from build123d import *

# Parameters (mm, degrees)
SKETCH1_W                = 170
SKETCH1_H                = 100
BOSS_EXTRUDE1_DEPTH      = 15
SKETCH2_W                = 70
SKETCH2_H                = 70
CUT_EXTRUDE1_DEPTH       = 13
SKETCH3_W                = 70
SKETCH3_H                = 90
CUT_EXTRUDE2_DEPTH       = 12
SKETCH8_W                = 15
SKETCH8_H                = 15
CUT_EXTRUDE9_DEPTH       = 2.5
SKETCH9_W                = 15
SKETCH9_H                = 15
CUT_EXTRUDE10_DEPTH      = 2.5
SKETCH10_W               = 12
SKETCH10_H               = 90
CUT_EXTRUDE11_DEPTH      = 10
SKETCH11_W               = 80
SKETCH11_H               = 90
BOSS_EXTRUDE2_DEPTH      = 10
SKETCH12_W               = 22
SKETCH12_H               = 90
BOSS_EXTRUDE4_DEPTH      = 4
SKETCH2_2_W              = 70
SKETCH2_2_H              = 70
CUT_EXTRUDE12_DEPTH      = 22
SKETCH13_W               = 74
SKETCH13_H               = 74
SKETCH13_W_2             = 70
SKETCH13_H_2             = 70
CUT_EXTRUDE13_DEPTH      = 4
BOSS_EXTRUDE6_DEPTH      = 100
SKETCH15_W               = 5
SKETCH15_H               = 3
CUT_EXTRUDE14_DEPTH      = 15
SKETCH16_R               = 4
SKETCH16_R_2             = 3
BOSS_EXTRUDE7_DEPTH      = 15
SKETCH16_3_R             = 3
CUT_EXTRUDE15_DEPTH      = 15
FILLET1_R                = 2
CUT_EXTRUDE16_DEPTH      = 145.387791679
CUT_EXTRUDE16_DEPTH_BACK = 15


with BuildPart() as part:
    # Sketch1 → Boss-Extrude1 (new body)
    with BuildSketch(Plane.XY):
        with Locations((-16.108033241, 2.077562327)):
            Rectangle(SKETCH1_W, SKETCH1_H)
    extrude(amount=BOSS_EXTRUDE1_DEPTH)

    # Sketch2 → Cut-Extrude1 (cut)
    with BuildSketch(Plane(origin=(0, 0, 0), x_dir=(-1, 0, 0), z_dir=(0, 0, -1))):
        with Locations((-23.891966759, 2.077562327)):
            Rectangle(SKETCH2_W, SKETCH2_H)
    extrude(amount=-CUT_EXTRUDE1_DEPTH, mode=Mode.SUBTRACT)

    # Sketch3 → Cut-Extrude2 (cut)
    with BuildSketch(Plane.XY.offset(15)):
        with Locations((-56.108033241, 2.077562327)):
            Rectangle(SKETCH3_W, SKETCH3_H)
    extrude(amount=-CUT_EXTRUDE2_DEPTH, mode=Mode.SUBTRACT)

    # Sketch8 → Cut-Extrude9 (cut)
    with BuildSketch(Plane(origin=(0, 52.077562327, 0), x_dir=(1, 0, 0), z_dir=(0, 1, 0))):
        with Locations((-93.608033241, -7.5)):
            Rectangle(SKETCH8_W, SKETCH8_H)
    extrude(amount=-CUT_EXTRUDE9_DEPTH, mode=Mode.SUBTRACT)

    # Sketch9 → Cut-Extrude10 (cut)
    with BuildSketch(Plane.XZ.offset(47.922437673)):
        with Locations((-93.608033241, 7.5)):
            Rectangle(SKETCH9_W, SKETCH9_H)
    extrude(amount=-CUT_EXTRUDE10_DEPTH, mode=Mode.SUBTRACT)

    # Sketch10 → Cut-Extrude11 (cut)
    with BuildSketch(Plane.ZY.offset(21.108033241)):
        with Locations((9, 2.077562327)):
            Rectangle(SKETCH10_W, SKETCH10_H)
    extrude(amount=-CUT_EXTRUDE11_DEPTH, mode=Mode.SUBTRACT)

    # Sketch11 → Boss-Extrude2 (add)
    with BuildSketch(Plane.XY.offset(15)):
        Polygon((-86.108033241, -45.422437673), (-86.108033241, -47.922437673), (68.891966759, -47.922437673), (68.891966759, 52.077562327), (-86.108033241, 52.077562327), (-86.108033241, 49.577562327), (-101.108033241, 49.577562327), (-101.108033241, -45.422437673), align=None)
        with Locations((-51.108033241, 2.077562327)):
            Rectangle(SKETCH11_W, SKETCH11_H, mode=Mode.SUBTRACT)
    extrude(amount=BOSS_EXTRUDE2_DEPTH)

    # Sketch12 → Boss-Extrude4 (add)
    with BuildSketch(Plane.ZY.offset(11.108033241)):
        with Locations((14, 2.077562327)):
            Rectangle(SKETCH12_W, SKETCH12_H)
    extrude(amount=BOSS_EXTRUDE4_DEPTH)

    # Sketch2<2> → Cut-Extrude12 (cut)
    with BuildSketch(Plane(origin=(0, 0, 0), x_dir=(-1, 0, 0), z_dir=(0, 0, -1))):
        with Locations((-23.891966759, 2.077562327)):
            Rectangle(SKETCH2_2_W, SKETCH2_2_H)
    extrude(amount=-CUT_EXTRUDE12_DEPTH, mode=Mode.SUBTRACT)

    # Sketch13 → Cut-Extrude13 (cut)
    with BuildSketch(Plane(origin=(0, 0, 0), x_dir=(-1, 0, 0), z_dir=(0, 0, -1))):
        with Locations((-23.891966759, 2.077562327)):
            Rectangle(SKETCH13_W, SKETCH13_H)
        with Locations((-23.891966759, 2.077562327)):
            Rectangle(SKETCH13_W_2, SKETCH13_H_2, mode=Mode.SUBTRACT)
    extrude(amount=-CUT_EXTRUDE13_DEPTH, mode=Mode.SUBTRACT)

    # Sketch14 → Boss-Extrude6 (add)
    with BuildSketch(Plane(origin=(0, 52.077562327, 0), x_dir=(1, 0, 0), z_dir=(0, 1, 0))):
        Polygon((-86.108033241, 0), (-78.108033241, 0), (-86.108033241, 8), align=None)
    extrude(amount=-BOSS_EXTRUDE6_DEPTH)

    # Sketch15 → Cut-Extrude14 (cut)
    with BuildSketch(Plane.ZY.offset(101.108033241)):
        with Locations((12.5, 48.077562327)):
            Rectangle(SKETCH15_W, SKETCH15_H)
        with Locations((12.5, -43.922437673)):
            Rectangle(SKETCH15_W, SKETCH15_H)
    extrude(amount=-CUT_EXTRUDE14_DEPTH, mode=Mode.SUBTRACT)

    # Sketch16 → Boss-Extrude7 (add)
    with BuildSketch(Plane(origin=(-11.108033241, 0, 0), x_dir=(0, 0, -1), z_dir=(1, 0, 0))):
        with Locations(Location((-15.920102605, 0, 0), (0, 0, 90))):
            Circle(SKETCH16_R)
        with Locations(Location((-15.920102605, 0, 0), (0, 0, 90))):
            Circle(SKETCH16_R_2, mode=Mode.SUBTRACT)
    extrude(amount=-BOSS_EXTRUDE7_DEPTH)

    # Sketch16<3> → Cut-Extrude15 (cut)
    with BuildSketch(Plane(origin=(-11.108033241, 0, 0), x_dir=(0, 0, -1), z_dir=(1, 0, 0))):
        with Locations(Location((-15.920102605, 0, 0), (0, 0, 90))):
            Circle(SKETCH16_3_R)
    extrude(amount=-CUT_EXTRUDE15_DEPTH, mode=Mode.SUBTRACT)

    # Fillet1
    # the kernel refuses this fillet: 2 mm, written as the material it takes off along each edge
    with BuildSketch(Plane(origin=(-26.108033241, 0, 15.920102605), x_dir=(0, 1, 0), z_dir=(0, 0, -1))) as fillet1_piece_1:
        with BuildLine():
            CenterArc((2, 1.732050808), FILLET1_R, 300, 60)
            Line((3, 0), (3.02, -0.034641016))
            ThreePointArc((3.02, -0.034641016), (3.5, -0.04), (4, -0.04))
            Line((4, -0.04), (4.04, 0))
            Line((4.04, 0), (4.04, 1.732050808))
            Line((4.04, 1.732050808), (4, 1.732050808))
        make_face()
    revolve(axis=Axis((-26.108033241, 0, 15.920102605), (1, 0, 0)), mode=Mode.SUBTRACT)

    # Sketch17 → Cut-Extrude16 (cut, two sides: drawn at the far end of the back side and taken through both)
    with BuildSketch(Plane(origin=(0, 52.077562327, 0), x_dir=(1, 0, 0), z_dir=(0, 1, 0)).offset(-CUT_EXTRUDE16_DEPTH_BACK)):
        with BuildLine():
            Line((-64.771644572, -25), (-64.771644572, -19.506214928))
            ThreePointArc((-64.771644572, -19.506214928), (-69.270802051, -15.007057449), (-73.76995953, -19.506214928))
            Line((-73.76995953, -19.506214928), (-73.76995953, -25))
            Line((-73.76995953, -25), (-64.771644572, -25))
        make_face()
    extrude(amount=CUT_EXTRUDE16_DEPTH + CUT_EXTRUDE16_DEPTH_BACK, mode=Mode.SUBTRACT)


solid = part.part
Part model, mm, in its own coordinate system. A direction names the side the tool comes from. Give positions to 0.01 mm unless a question says otherwise; leave off trailing zeros. Write each loop counter-clockwise with the first axis right and the second up, starting at its lowest first coordinate (ties: lowest second). Pieces come first, ordered by that corner, then holes.
1) Probe L1, parallel to X at y = 32.5, z = 18.5; L2, parallel to Z at x = -20, y = 0; L3, parallel to Y at x = 34, z = 6.5. List the from-to ranges inside material, lowest first.
Resolved:
L1: x = -101.11 to -91.11, -15.11 to -11.11, 58.89 to 68.89
L2: z = 0 to 3, 11.92 to 12.92, 18.92 to 19.92
L3: y = -47.92 to -32.92, 37.08 to 52.08
2) Cut at C-C on x = -81. Write the cut outline in (y, z), then the cut area to 3 significant figures.
Resolved:
outline: (-47.92, -2.89) - (52.08, -2.89) - (52.08, 25) - (47.08, 25) - (47.08, 3) - (-42.92, 3) - (-42.92, 25) - (-47.92, 25) - close
area: 809 mm2
3) Cut at A-A on x = 24. Write the cut outline in (y, z), then the cut area to 3 significant figures.
Resolved:
outline: (-47.92, 0) - (-34.92, 0) - (-34.92, 4) - (-32.92, 4) - (-32.92, 22) - (37.08, 22) - (37.08, 4) - (39.08, 4) - (39.08, 0) - (52.08, 0) - (52.08, 25) - (-47.92, 25) - close
area: 944 mm2
4) Cut at D-D on x = -56. Write the cut outline in (y, z), then the cut area to 3 significant figures.
Resolved:
outline: (-47.92, 0) - (52.08, 0) - (52.08, 25) - (47.08, 25) - (47.08, 3) - (-42.92, 3) - (-42.92, 25) - (-47.92, 25) - close
area: 520 mm2
5) Which spindle directions (+Z, -Z, +X, -X, +Y, -Y) get a long thin tool onto all of the face, cutting with end or side? Do faces 1 (the face through (-94, -45.422, 5)), 2 (the face through (24, -34.922, 2)), 3 (the face through (-54, 47.078, 14)). Say none if no direction does.
Resolved:
face 1: +Z, -Z, -X, -Y
face 2: -Z
face 3: +Z
6) Two-plate mould, pull along X, no slides. Class faces 4 (the face through (-19.677, -0.867, 12.015)), 5 (the face through (68.892, 1, 12)), 6 (the face through (26.8, -33.4, 4)), 7 (the face through (-94, 48, 10)): released by +X, released by -X, zero draft, split by the parting line, or undercut.
Resolved:
face 4: undercut
face 5: released by +X
face 6: undercut
face 7: zero draft
7) Cut at B-B on y = -31. Write the cut outline in (x, z).
Resolved:
outline: (-101.11, 0) - (-86.11, 0) - (-86.11, -8) - (-78.11, 0) - (-13.11, 0) - (-13.11, 4) - (-11.11, 4) - (-11.11, 22) - (58.89, 22) - (58.89, 4) - (60.89, 4) - (60.89, 0) - (68.89, 0) - (68.89, 25) - (-15.11, 25) - (-15.11, 3) - (-91.11, 3) - (-91.11, 25) - (-101.11, 25) - close
8) Pin check, flat tips, straight feed: pin 1 (3 mm diameter, centred on x = 16.5, y = 2.5, fed in from -Z); pin 2 (10 mm diameter, centred on x = -64, y = 26, fed in from +Z); pin 3 (5 mm diameter, centred on x = -97, z = 21.5, fed in from -Y). Stop position of each tip, or through.
Resolved:
pin 1: stops at z = 22
pin 2: stops at z = 3
pin 3: stops at y = -45.42
